Model file for the job. Use its own axes, mm. A direction names the side the tool comes from. Give positions to 0.01 mm unless a question says otherwise; leave off trailing zeros. Loops run counter-clockwise (first coordinate to the right, second up) from the corner with the lowest first, then second, coordinate; pieces in that order, holes last. Notation, with made-up numbers: (52, 41.25) -> (74, 41.25) arc R24 cw to (74, 59.25) -> close; hole circle Ø7 at (-30.5, 1). An arc over 180 degrees is marked (long way). Use CSV: the item, a comma, the result in double quotes. Start each with the question number.
(1) 3-axis set-ups, long thin cutter, end or side, ignore diameter. For faces 1 (the flat face through (-39.2, 1609.9, -1628.4)), 2 (the flat face through (-20, 1629.5, -813)): which of +Z, -Z, +X, -X, +Y, -Y reach the whole face in a straight line?
(2) Cut at C-C on z = -240. Write the cut outline in (x, y).
(3) Cut at B-B on x = -20.5. Write the cut outline in (y, z), then the cut area to 3 significant figures.
(4) Cut at A-A on y = 1601.5. Write the cut outline in (x, z), then the cut area to 3 significant figures.
(5) Drill centre lines: probe 1 along X at (y, z) = (1623.5, -989); probe 2 along Y at (x, z) = (-36, -350). Where is each one in solid material? Low to high.
(6) Pull direction Y, two halves, no side cores. Call faces 3 (the flat face through (-2, 1611, -813)), 4 (the flat face through (-20, 1593.5, -814)), 5 (the flat face through (-20, 1631.5, -813)), 6 (the flat face through (-40, 1611, -813)): pulls with the +Y half, pulls with the -Y half, needs draft (parallel to the pull), parting line crosses it, or undercut.
from build123d import *

# Parameters (mm, degrees)
SKETCH1_W           = 40
SKETCH1_H           = 40
SKETCH1_W_2         = 36
SKETCH1_H_2         = 36
BOSS_EXTRUDE1_DEPTH = 1650
CUT_EXTRUDE1_REACH  = 2322.753


with BuildPart() as part:
    # Sketch1 → Boss-Extrude1 (new body)
    with BuildSketch(Plane.XY):
        with Locations((-20, 1611.5)):
            Rectangle(SKETCH1_W, SKETCH1_H)
        with Locations((-20, 1611.5)):
            Rectangle(SKETCH1_W_2, SKETCH1_H_2, mode=Mode.SUBTRACT)
    extrude(amount=-BOSS_EXTRUDE1_DEPTH)

    # Cut-Extrude1: up to this face of the body (flat: up to its plane)
    cut_extrude1_end = Plane(part.part.faces().sort_by_distance((-40, 1611.5, -825))[0])
    # Sketch2 → Cut-Extrude1 (cut, up to the picked face)
    with BuildSketch(Plane(origin=(0, 0, 0), x_dir=(0, 0, -1), z_dir=(1, 0, 0)), mode=Mode.PRIVATE) as cut_extrude1_sk1:
        Polygon((0, 1631.5), (0, 1591.5), (40, 1591.5), align=None)
    cut_extrude1_tool1 = split(extrude(cut_extrude1_sk1.sketch, amount=-CUT_EXTRUDE1_REACH, mode=Mode.PRIVATE), bisect_by=cut_extrude1_end, keep=Keep.BOTH, mode=Mode.PRIVATE)
    # Sketch2 → Cut-Extrude1 (cut, up to the picked face)
    with BuildSketch(Plane(origin=(0, 0, 0), x_dir=(0, 0, -1), z_dir=(1, 0, 0)), mode=Mode.PRIVATE) as cut_extrude1_sk2:
        Polygon((1610, 1591.5), (1650, 1631.5), (1650, 1591.5), align=None)
    cut_extrude1_tool2 = split(extrude(cut_extrude1_sk2.sketch, amount=-CUT_EXTRUDE1_REACH, mode=Mode.PRIVATE), bisect_by=cut_extrude1_end, keep=Keep.BOTH, mode=Mode.PRIVATE)
    add(cut_extrude1_tool1.solids().sort_by(Axis((0, 1604.833333, -13.333333), (-1, 0, 0)))[0], mode=Mode.SUBTRACT)
    add(cut_extrude1_tool2.solids().sort_by(Axis((0, 1604.833333, -1636.666667), (-1, 0, 0)))[0], mode=Mode.SUBTRACT)


solid = part.part
Check result:
1,face 1,"-Z, +X, -X, -Y"
1,face 2,"+Z, -Z"
2,outline,"(-40, 1591.5) -> (0, 1591.5) -> (0, 1631.5) -> (-40, 1631.5) -> close; hole (-38, 1593.5) -> (-2, 1593.5) -> (-2, 1629.5) -> (-38, 1629.5) -> close"
3,outline,"(1591.5, -1610) -> (1593.5, -1612) -> (1593.5, -38) -> (1591.5, -40) -> close; (1629.5, -1648) -> (1631.5, -1650) -> (1631.5, 0) -> (1629.5, -2) -> close"
3,area,"6,440 mm²"
4,outline,"(-40, -1620) -> (-38, -1620) -> (-38, -30) -> (-40, -30) -> close; (-2, -1620) -> (0, -1620) -> (0, -30) -> (-2, -30) -> close"
4,area,"6,360 mm²"
5,probe 1,"-40 to -38, -2 to 0"
5,probe 2,"1591.5 to 1593.5, 1629.5 to 1631.5"
6,face 3,"undercut"
6,face 4,"undercut"
6,face 5,"pulls with the +Y half"
6,face 6,"needs draft"
